Drawing for the job (mm, zero at the part's lowest x, y, z). A direction names the side the tool comes from. Coordinates: 2 decimals unless noted, no trailing zeros. Write each loop counter-clockwise with the first axis right and the second up, starting at its lowest first coordinate (ties: lowest second). Pieces come first, ordered by that corner, then holes. Notation, with made-up numbers: M 19.25,63.25 L 46.25,63.25 A25 ccw 46.25,95.25 Z; hole C 52.25,75 d7. An arc over 180 degrees is marked long. Use a Markdown table: item, result. Add a question column.
Q1. Slice it at D-D on z = 15.5. Write the cut outline in (x, y), then the cut area to 4 significant figures.
Q2. Pin check, flat tips, straight feed: pin 1 Ø8 at (x, z) = (8.5, 15.5) entering from +Y; pin 2 Ø3 at (x, z) = (3.5, 17) entering from -Y; pin 3 Ø2 at (x, z) = (6, 15.5) entering from -Y. Stop position of each tip, or through.
Q3. Mould opens along X. For the marked faces 3, 4 and 5 say: released by +X, released by -X, zero draft, split by the parting line, or undercut.
Q4. Tool access for the marked faces 1 and 2: list every direction of +Z, -Z, +X, -X, +Y, -Y with a clear straight run to the whole face (end or side of a thin tool).
Q5. Wall check: L1, parallel to Y at x = 1, z = 1.5; L2, parallel to Y at x = 6.25, z = 6.5; L3, parallel to Z at x = 8.5, y = 26.5. Give the ranges that are in metal, low to high. Write a range as from..to.
Q6. Slice it at C-C on y = 21. Write the cut outline in (x, z).
Q7. Slice it at A-A on x = 8.5. Write the cut outline in (y, z).
Q8. Slice it at B-B on z = 6. Write the cut outline in (x, y).
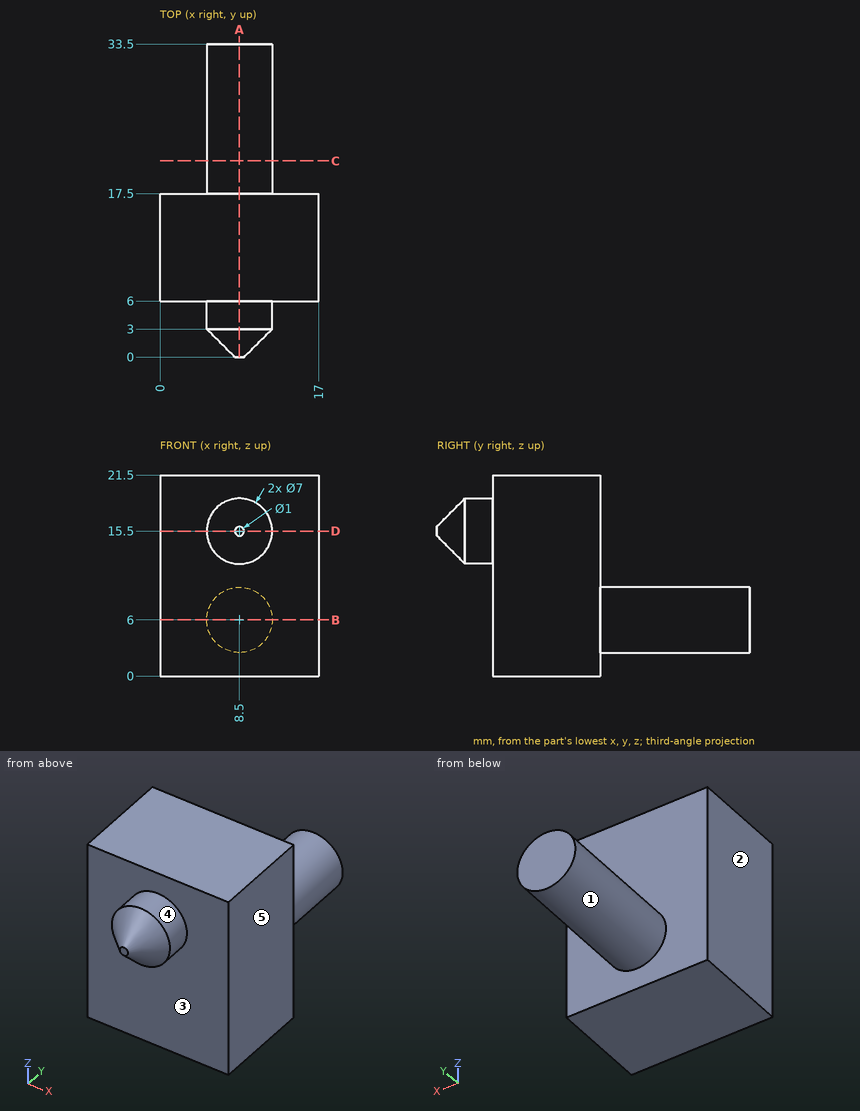
Recorded:
| question | item | result |
|---|---|---|
| 1 | outline | M 0,6 L 5,6 L 5,3 L 8,0 L 9,0 L 12,3 L 12,6 L 17,6 L 17,17.5 L 0,17.5 Z |
| 1 | area | 228.5 mm² |
| 2 | pin 1 | y = 17.5 |
| 2 | pin 2 | y = 6 |
| 2 | pin 3 | y = 1 |
| 3 | face 3 | zero draft |
| 3 | face 4 | split by the parting line |
| 3 | face 5 | released by +X |
| 4 | face 1 | +Y |
| 4 | face 2 | +Z, -Z, -X, +Y, -Y |
| 5 | L1 | 6..17.5 |
| 5 | L2 | 6..33.5 |
| 5 | L3 | 2.5..9.5 |
| 6 | outline | C 8.5,6 d7 |
| 7 | outline | M 0,15 L 3,12 L 6,12 L 6,0 L 17.5,0 L 17.5,2.5 L 33.5,2.5 L 33.5,9.5 L 17.5,9.5 L 17.5,21.5 L 6,21.5 L 6,19 L 3,19 L 0,16 Z |
| 8 | outline | M 0,6 L 17,6 L 17,17.5 L 12,17.5 L 12,33.5 L 5,33.5 L 5,17.5 L 0,17.5 Z |
